Part print with two shaded views. Sizes in mm from the minimum x, y, z corner. A direction names the side the tool comes from. Give positions to 0.01 mm unless a question says otherwise; leave off trailing zeros. Write each loop counter-clockwise with the first axis right and the second up, starting at its lowest first coordinate (ties: lowest second). Pieces come first, ordered by that corner, then holes.
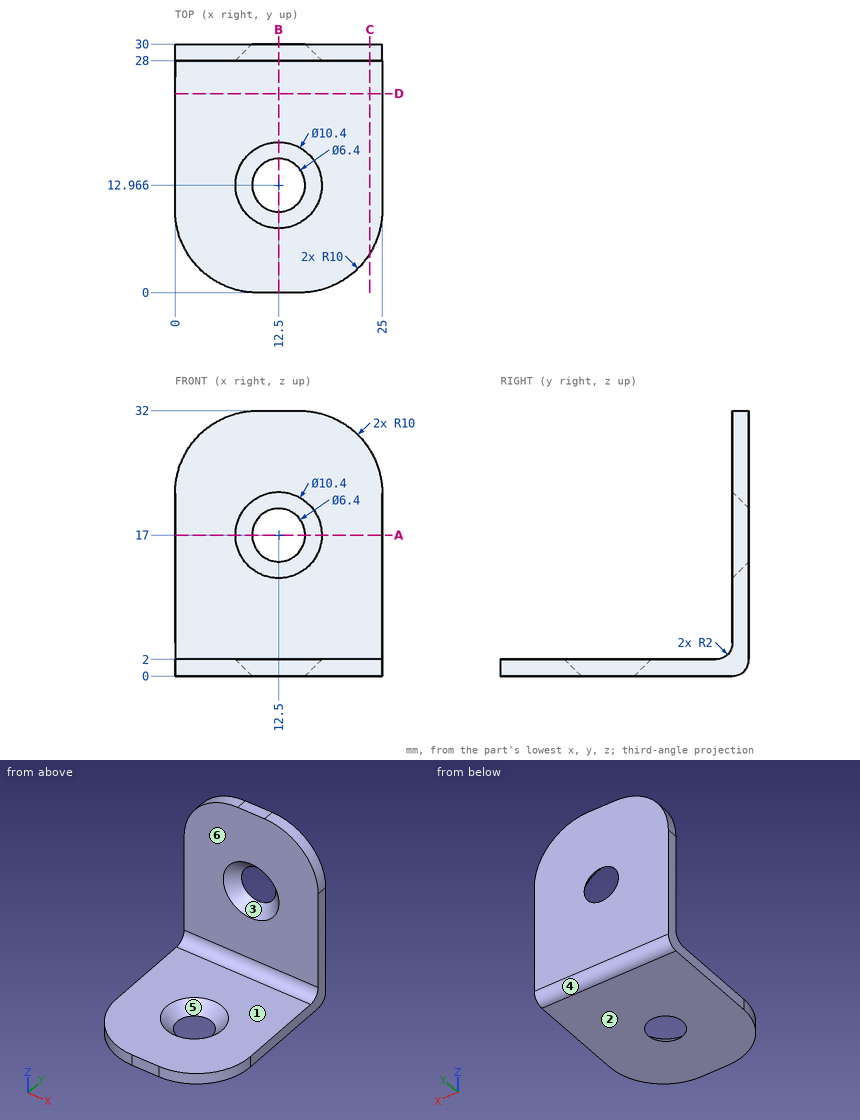
1) Flat gauge pin, fed straight in: P1, Ø12, axis at x = 10, z = 25.5, coming from the -Y side. Where does the tip first touch, or does it go through?
Check result:
P1: stops at y = 28
2) Drill centre lines: L1, parallel to Y at x = 4, z = 28; L2, parallel to Z at x = 23, y = 17; L3, parallel to Y at x = 14, z = 20.5. Where is each one in solid material? Low to high.
Check result:
L1: y = 28 to 30
L2: z = 0 to 2
L3: y = 29.39 to 30
3) Saw through at A-A (z = 17). Write the cut outline in (x, y).
Check result:
outline: (0, 28) - (7.3, 28) - (9.3, 30) - (0, 30) - close; (15.7, 30) - (17.7, 28) - (25, 28) - (25, 30) - close
4) Mould opens along Z. For the marked faces 3, 4, 5 and 6 say: +Z half, -Z half, draft (parallel to the pull), parting line (faces both ways), or undercut.
Check result:
face 3: undercut
face 4: -Z half
face 5: +Z half
face 6: draft
5) Saw through at D-D (y = 24). Write the cut outline in (x, z).
Check result:
outline: (0, 0) - (25, 0) - (25, 2) - (0, 2) - close
6) 3-axis set-ups, long thin cutter, end or side, ignore diameter. For the marked faces 1 and 2: which of +Z, -Z, +X, -X, +Y, -Y reach the whole face in a straight line?
Check result:
face 1: +Z, +X, -X, -Y
face 2: -Z, +X, -X, +Y, -Y
7) Saw through at B-B (x = 12.5). Write the cut outline in (y, z), and give its area (3 significant figures).
Check result:
outline: (0, 0) - (9.77, 0) - (7.77, 2) - (0, 2) - close; (16.17, 0) - (28, 0) arc R2 ccw to (30, 2) - (30, 13.8) - (28, 11.8) - (28, 4) arc R2 cw to (26, 2) - (18.17, 2) - close; (28, 22.2) - (30, 20.2) - (30, 32) - (28, 32) - close
area: 86.4 mm2
8) Saw through at C-C (x = 23.5). Write the cut outline in (y, z).
Check result:
outline: (4.73, 0) - (28, 0) arc R2 ccw to (30, 2) - (30, 27.27) - (28, 27.27) - (28, 4) arc R2 cw to (26, 2) - (4.73, 2) - close
